Study the drawing (mm; zero at the part's minimum x, y, z) and answer. A direction names the side the tool comes from. Give positions to 0.01 mm unless a question says otherwise; leave off trailing zeros. Write each loop counter-clockwise with the first axis right and the second up, starting at its lowest first coordinate (ties: lowest second). Pieces come first, ordered by that corner, then holes. Notation, with made-up numbers: (-37.5, 76.5) -> (1.5, 76.5) arc R10 ccw to (1.5, 92.5) -> close; hole circle Ø10 at (6, -31). An arc over 180 degrees is marked (long way). Put each result on its own line as item: value. Start each with the question number.
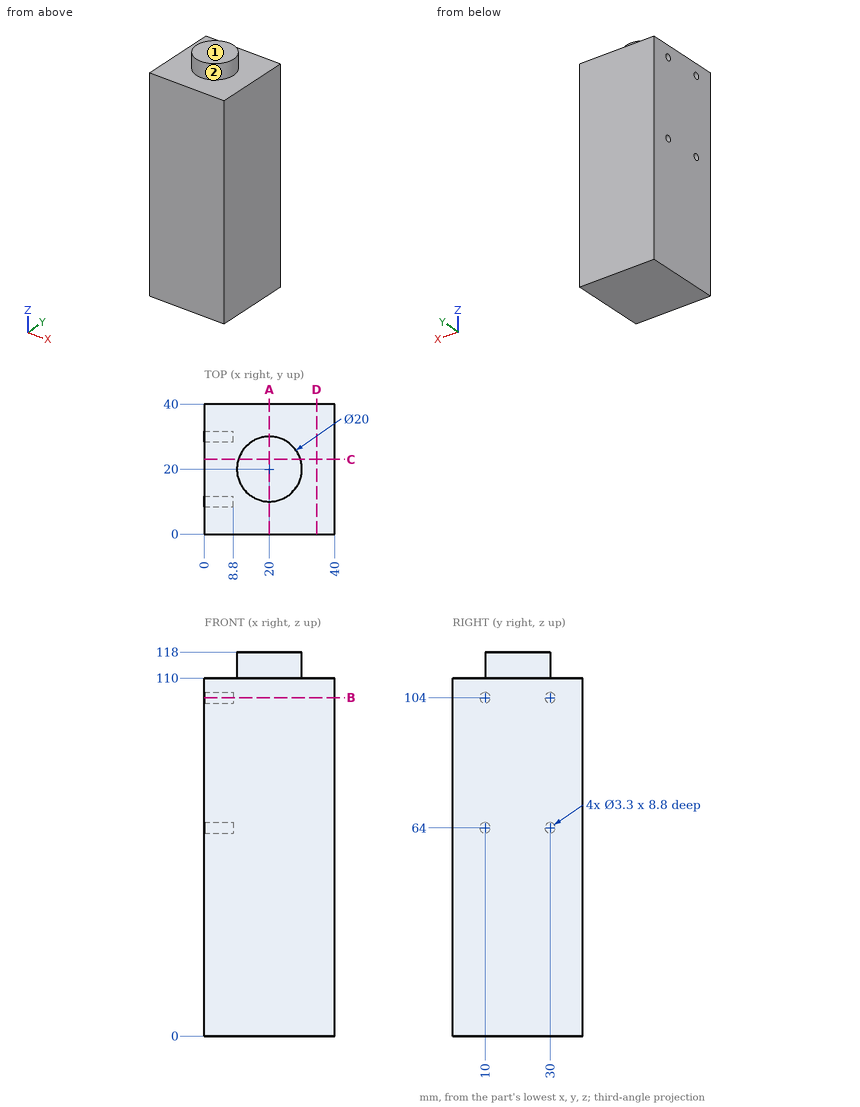
1) A cutting plane is placed at D-D on x = 34.5. Give the vertices of the cut face in (y, z), and give its area (3 significant figures).
2) A cutting plane is placed at B-B on z = 104. Give the vertices of the cut face in (x, y).
3) A cutting plane is placed at C-C on y = 23. Give the vertices of the cut face in (x, z).
4) This flat-tipped pin is pushed along its axis until it touches: pin 1 Ø1 at (y, z) = (9.5, 64.5) entering from -X. Where does it stop, or does it pass through?
5) Straight lines are drawn through the part: line 1 (Y direction, x = 2, z = 64); line 2 (Z direction, x = 5, y = 10); line 3 (Z direction, x = 5.5, y = 16). For each, find the intervals that lie inside material, in ascending order. Write a range as [from, to].
6) For the marked faces 1 and 2, determine the directions among +Z, -Z, +X, -X, +Y, -Y from which every point of the face is accessible in a straight line to the end or side of a thin tool.
7) A cutting plane is placed at A-A on x = 20. Give the vertices of the cut face in (y, z).
Results found:
1. outline: (0, 0) -> (40, 0) -> (40, 110) -> (0, 110) -> close
1. area: 4,400 mm²
2. outline: (0, 0) -> (40, 0) -> (40, 40) -> (0, 40) -> (0, 31.65) -> (8.8, 31.65) -> (8.8, 28.35) -> (0, 28.35) -> (0, 11.65) -> (8.8, 11.65) -> (8.8, 8.35) -> (0, 8.35) -> close
3. outline: (0, 0) -> (40, 0) -> (40, 110) -> (29.54, 110) -> (29.54, 118) -> (10.46, 118) -> (10.46, 110) -> (0, 110) -> close
4. pin 1: stops at x = 8.8
5. line 1: y = [0, 8.35], [11.65, 28.35], [31.65, 40]
5. line 2: z = [0, 62.35], [65.65, 102.35], [105.65, 110]
5. line 3: z = [0, 110]
6. face 1: +Z, +X, -X, +Y, -Y
6. face 2: +Z
7. outline: (0, 0) -> (40, 0) -> (40, 110) -> (30, 110) -> (30, 118) -> (10, 118) -> (10, 110) -> (0, 110) -> close
